```python
from build123d import *

# Parameters (mm, degrees)
BOSS_EXTRUDE1_DEPTH                                  = 300
SKETCH2_R                                            = 30
CUT_EXTRUDE1_DEPTH                                   = 319.198051534
SKETCH3_W                                            = 40
SKETCH3_H                                            = 56
CUT_EXTRUDE2_DEPTH                                   = 10
SKETCH4_W                                            = 40
SKETCH4_H                                            = 52
CUT_EXTRUDE3_DEPTH                                   = 10
FILLET1_R                                            = 3
CSK_FOR_M10_COUNTERSUNK_FLAT_HEAD_SCREW1_D           = 11
CSK_FOR_M10_COUNTERSUNK_FLAT_HEAD_SCREW1_DEPTH       = 20.003
CSK_FOR_M10_COUNTERSUNK_FLAT_HEAD_SCREW1_CSINK_D     = 20
CSK_FOR_M10_COUNTERSUNK_FLAT_HEAD_SCREW1_CSINK_ANGLE = 90
CSK_FOR_M10_COUNTERSUNK_FLAT_HEAD_SCREW1_TIP         = 3.304733405


with BuildPart() as part:
    # Sketch1 → Boss-Extrude1 (new body)
    with BuildSketch(Plane.XY):
        Polygon((0, -37.5), (0, 37.5), (75, 37.5), (75, 31.15), (6.35, 31.15), (6.35, -31.15), (75, -31.15), (75, -37.5), align=None)
    extrude(amount=BOSS_EXTRUDE1_DEPTH)

    # Sketch2 → Cut-Extrude1 (cut, through all)
    with BuildSketch(Plane(origin=(0, 37.5, 0), x_dir=(1, 0, 0), z_dir=(0, 1, 0))):
        with Locations(Location((40, -150, 0), (0, 0, 270))):
            Circle(SKETCH2_R)
    extrude(amount=-CUT_EXTRUDE1_DEPTH, mode=Mode.SUBTRACT)

    # Sketch3 → Cut-Extrude2 (cut)
    with BuildSketch(Plane.XZ.offset(37.5)):
        with Locations((40, 63)):
            Rectangle(SKETCH3_W, SKETCH3_H)
    extrude(amount=-CUT_EXTRUDE2_DEPTH, mode=Mode.SUBTRACT)

    # Sketch4 → Cut-Extrude3 (cut)
    with BuildSketch(Plane(origin=(0, 37.5, 0), x_dir=(1, 0, 0), z_dir=(0, 1, 0))):
        with Locations((40, -84)):
            Rectangle(SKETCH4_W, SKETCH4_H)
    extrude(amount=-CUT_EXTRUDE3_DEPTH, mode=Mode.SUBTRACT)

    # Fillet1
    fillet1_edges = [part.edges().sort_by_distance(p)[0] for p in [
        (20, -34.325, 91),
        (60, -34.325, 91),
        (60, -34.325, 35),
        (20, -34.325, 35),
        (60, 34.325, 110),
        (20, 34.325, 110),
        (20, 34.325, 58),
        (60, 34.325, 58),
    ]]
    fillet(fillet1_edges, radius=FILLET1_R)

    # CSK for M10 Countersunk Flat Head Screw1
    with Locations(Plane.ZY):
        with Locations((74.704121605, 1.01110333), (72.25, -20.6), (79.836004025, 23.188381743)):
            CounterSinkHole(CSK_FOR_M10_COUNTERSUNK_FLAT_HEAD_SCREW1_D / 2, CSK_FOR_M10_COUNTERSUNK_FLAT_HEAD_SCREW1_CSINK_D / 2, depth=CSK_FOR_M10_COUNTERSUNK_FLAT_HEAD_SCREW1_DEPTH, counter_sink_angle=CSK_FOR_M10_COUNTERSUNK_FLAT_HEAD_SCREW1_CSINK_ANGLE)
            with Locations((0, 0, -(CSK_FOR_M10_COUNTERSUNK_FLAT_HEAD_SCREW1_DEPTH + CSK_FOR_M10_COUNTERSUNK_FLAT_HEAD_SCREW1_TIP / 2))):  # 118° drill point
                Cone(0, CSK_FOR_M10_COUNTERSUNK_FLAT_HEAD_SCREW1_D / 2, CSK_FOR_M10_COUNTERSUNK_FLAT_HEAD_SCREW1_TIP, mode=Mode.SUBTRACT)


solid = part.part
```
The listing builds one solid part. Answer for the finished solid, in the listing's coordinates (mm). A direction names the side the tool comes from. Round coordinates to 2 decimals unless told otherwise and drop trailing zeros. Loops run counter-clockwise (first coordinate to the right, second up) from the corner with the lowest first, then second, coordinate; pieces in that order, holes last.
1) A cutting plane is placed at D-D on x = 54. Determine the outline of the cut face in (y, z).
Outcome:
outline: (-37.5, 0) - (-31.15, 0) - (-31.15, 35) - (-37.5, 35) - close; (-37.5, 91) - (-31.15, 91) - (-31.15, 123.47) - (-37.5, 123.47) - close; (-37.5, 176.53) - (-31.15, 176.53) - (-31.15, 300) - (-37.5, 300) - close; (31.15, 0) - (37.5, 0) - (37.5, 58) - (31.15, 58) - close; (31.15, 110) - (37.5, 110) - (37.5, 123.47) - (31.15, 123.47) - close; (31.15, 176.53) - (37.5, 176.53) - (37.5, 300) - (31.15, 300) - close
2) A cutting plane is placed at A-A on x = 40. Determine the outline of the cut face in (y, z), plus the area to 3 significant figures.
Outcome:
outline: (-37.5, 0) - (-31.15, 0) - (-31.15, 35) - (-37.5, 35) - close; (-37.5, 91) - (-31.15, 91) - (-31.15, 120) - (-37.5, 120) - close; (-37.5, 180) - (-31.15, 180) - (-31.15, 300) - (-37.5, 300) - close; (31.15, 0) - (37.5, 0) - (37.5, 58) - (31.15, 58) - close; (31.15, 110) - (37.5, 110) - (37.5, 120) - (31.15, 120) - close; (31.15, 180) - (37.5, 180) - (37.5, 300) - (31.15, 300) - close
area: 2,360 mm2
3) A cutting plane is placed at C-C on z = 150. Determine the outline of the cut face in (x, y).
Outcome:
outline: (0, -37.5) - (10, -37.5) - (10, -31.15) - (6.35, -31.15) - (6.35, 31.15) - (10, 31.15) - (10, 37.5) - (0, 37.5) - close; (70, -37.5) - (75, -37.5) - (75, -31.15) - (70, -31.15) - close; (70, 31.15) - (75, 31.15) - (75, 37.5) - (70, 37.5) - close
4) A cutting plane is placed at B-B on z = 43.5. Determine the outline of the cut face in (x, y).
Outcome:
outline: (0, -37.5) - (20, -37.5) - (20, -31.15) - (6.35, -31.15) - (6.35, 31.15) - (75, 31.15) - (75, 37.5) - (0, 37.5) - close; (60, -37.5) - (75, -37.5) - (75, -31.15) - (60, -31.15) - close
5) For a pull along X with two mould halves and no side action, classify faces 4 (the face through (75, -34, 148)), 5 (the face through (4.28, 1.26, 80.42)), 6 (the face through (40, 34, 58)), 7 (the face through (5.438, -20.358, 77.745)) as released by +X, released by -X, zero draft, split by the parting line, or undercut.
Outcome:
face 4: released by +X
face 5: released by -X
face 6: undercut
face 7: zero draft
6) Consider line 1 (Y direction, x = 52.5, z = 180); line 2 (X direction, y = -34.5, z = 150); line 3 (X direction, y = 32, z = 74.5). Determine where each line is inside the solid, lowest interval first.
Outcome:
line 1: y = -37.5 to -31.15, 31.15 to 37.5
line 2: x = 0 to 10, 70 to 75
line 3: x = 0 to 20, 60 to 75
7) Given P1, Ø6, axis at x = 19.5, y = 27, coming from the -Z side; P2, Ø6, axis at y = -1.5, z = 81, coming from the +X side; P3, Ø14.5, axis at y = 23.19, z = 79.84, coming from the -X side, each flat-ended and moving along its own axis, determine where each tip first touches the part or whether it passes through.
Outcome:
P1: passes through
P2: stops at x = 6.35
P3: stops at x = 2.75
8) For faces 1 (the face through (40, -34, 35)), 2 (the face through (6.35, 0, 148)), 3 (the face through (20, 34, 84)), determine the directions among +Z, -Z, +X, -X, +Y, -Y from which every point of the face is accessible in a straight line to the end or side of a thin tool.
Outcome:
face 1: -Y
face 2: +Z, -Z, +X
face 3: +Y
